Source: CAD feature listing. Evaluate the final solid. Frame: model axes, mm. A direction names the side the tool comes from. Round coordinates to 2 decimals unless told otherwise and drop trailing zeros. Write each loop counter-clockwise with the first axis right and the second up, starting at its lowest first coordinate (ties: lowest second). Pieces come first, ordered by that corner, then holes. Notation, with made-up numbers: M 73,19.5 L 121,19.5 A23 cw 121,31.5 Z; hole C 56,-17 d2. An arc over 180 degrees is marked long. Use a Markdown table: item, result.
```python
from build123d import *

# Parameters (mm, degrees)
SKETCH1_R           = 88.9
SKETCH1_R_2         = 6
SKETCH1_R_3         = 6.35
BOSS_EXTRUDE1_DEPTH = 5
SKETCH2_R           = 6.35
BOSS_EXTRUDE2_DEPTH = 15


with BuildPart() as part:
    # Sketch1 → Boss-Extrude1 (new body)
    with BuildSketch(Plane.XY):
        Circle(SKETCH1_R)
        Circle(SKETCH1_R_2, mode=Mode.SUBTRACT)
        with Locations((0, -76.2)):
            Circle(SKETCH1_R_3, mode=Mode.SUBTRACT)
        with Locations((0, 76.2)):
            Circle(SKETCH1_R_3, mode=Mode.SUBTRACT)
    extrude(amount=BOSS_EXTRUDE1_DEPTH)

    # Sketch2 → Boss-Extrude2 (add)
    with BuildSketch(Plane.XY):
        with Locations((0, -76.2)):
            Circle(SKETCH2_R)
        with Locations((0, 76.2)):
            Circle(SKETCH2_R)
    extrude(amount=BOSS_EXTRUDE2_DEPTH)


solid = part.part
```
Q1. First-contact query: pin 1 Ø4 at (x, z) = (-45.5, 2.5) entering from +Y; pin 2 Ø8 at (x, z) = (9, 11.5) entering from +Y; pin 3 Ø2 at (x, y) = (53, 20.5) entering from +Z. Flat tips, straight axial feed; report the tip coordinate or a pass-through.
Results are:
| item | result |
|---|---|
| pin 1 | y = 77.53 |
| pin 2 | y = 80.11 |
| pin 3 | z = 5 |
Q2. Reachability of faces 5 (the flat face through (-1, -19, 0)), 6 (the cylindrical face through (3.414, -70.846, 9.93)) from +Z, -Z, +X, -X, +Y, -Y: full face, straight path, thin tool, end or side. Return the list, or none.
Results are:
| item | result |
|---|---|
| face 5 | -Z, +X, -X, +Y, -Y |
| face 6 | +Z |
Q3. Section B-B on z = 8.25. Return loops of the section in (x, y).
Results are:
| item | result |
|---|---|
| outline | C 0,-76.2 d12.7; C 0,76.2 d12.7 |
Q4. Line query: L1, parallel to Y at x = 0, z = 1.7; L2, parallel to Z at x = -27, y = -80.5; L3, parallel to X at y = -77, z = 9.5. Output: solid intervals per line, ascending.
Results are:
| item | result |
|---|---|
| L1 | -88.9 to -6, 6 to 88.9 |
| L2 | 0 to 5 |
| L3 | -6.3 to 6.3 |
Q5. Mould query, pull axis Y, two halves, no side actions, for faces 1 (the cylindrical face through (-6, 0, 2)), 2 (the cylindrical face through (84.795, 26.703, 2.465)), 3 (the cylindrical face through (-1.38, 70, 9.93)), 4 (the flat face through (0, 76, 15)). Classes: +Y half, -Y half, draft (parallel to the pull), parting line (faces both ways), or undercut.
Results are:
| item | result |
|---|---|
| face 1 | undercut |
| face 2 | parting line |
| face 3 | undercut |
| face 4 | draft |
Q6. Section D-D on x = -25.5. Return loops of the section in (y, z).
Results are:
| item | result |
|---|---|
| outline | M -85.16,0 L 85.16,0 L 85.16,5 L -85.16,5 Z |
Q7. Section A-A on x = 0. Return loops of the section in (y, z).
Results are:
| item | result |
|---|---|
| outline | M -88.9,0 L -6,0 L -6,5 L -69.85,5 L -69.85,15 L -82.55,15 L -82.55,5 L -88.9,5 Z; M 6,0 L 88.9,0 L 88.9,5 L 82.55,5 L 82.55,15 L 69.85,15 L 69.85,5 L 6,5 Z |
Q8. Section C-C on y = -76.2. Return loops of the section in (x, z).
Results are:
| item | result |
|---|---|
| outline | M -45.79,0 L 45.79,0 L 45.79,5 L 6.35,5 L 6.35,15 L -6.35,15 L -6.35,5 L -45.79,5 Z |
